```python
from build123d import *

# Parameters (mm, degrees)
SKETCH003_W          = 7
SKETCH003_H          = 3
SKETCH004_W          = 7
SKETCH004_H          = 3
SKETCH005_W          = 7
SKETCH005_H          = 3
SKETCH006_W          = 7
SKETCH006_H          = 3
POCKET_DEPTH         = 6.001
POCKET_DEPTH_BACK    = -6.001
POCKET001_DEPTH      = 6.001
POCKET001_DEPTH_BACK = -6.001
POCKET002_DEPTH      = 6.001
POCKET002_DEPTH_BACK = -6.001


with BuildPart() as part:
    # AdditivePipe: sweep along a path in Sketch
    with BuildLine(Plane.XY) as additivepipe_path:
        Line((0, 0), (0, 144))
    # Sketch002 → AdditivePipe (sweep)
    with BuildSketch(Plane.XZ):
        Polygon((-20, 6), (-20, -6), (-16, -6), (-16, -3), (-9, -3), (-9, -6), (9, -6), (9, -3), (16, -3), (16, -6), (20, -6), (20, 6), (16, 6), (16, 3), (9, 3), (9, 6), (-9, 6), (-9, 3), (-16, 3), (-16, 6), align=None)
    sweep(path=additivepipe_path.line)

    # AdditivePipe001: sweep along a path in Sketch001
    with BuildLine(Plane.XY) as additivepipe001_path:
        Line((0, 0), (0, 12))
        ThreePointArc((0, 12), (11.467071, 41.510976), (20, 72))
        ThreePointArc((20, 72), (28.532929, 102.489024), (40, 132))
        Line((40, 132), (40, 144))
    # Sketch002 → AdditivePipe001 (sweep)
    with BuildSketch(Plane.XZ):
        Polygon((-20, 6), (-20, -6), (-16, -6), (-16, -3), (-9, -3), (-9, -6), (9, -6), (9, -3), (16, -3), (16, -6), (20, -6), (20, 6), (16, 6), (16, 3), (9, 3), (9, 6), (-9, 6), (-9, 3), (-16, 3), (-16, 6), align=None)
    sweep(path=additivepipe001_path.line)

    # SubtractivePipe: sweep along a path in Sketch
    with BuildLine(Plane.XY) as subtractivepipe_path:
        Line((0, 0), (0, 144))
    # Sketch003 → SubtractivePipe (sweep, cut)
    with BuildSketch(Plane.XZ):
        with Locations((-12.5, 4.5)):
            Rectangle(SKETCH003_W, SKETCH003_H)
    sweep(path=subtractivepipe_path.line, mode=Mode.SUBTRACT)

    # SubtractivePipe001: sweep along a path in Sketch001
    with BuildLine(Plane.XY) as subtractivepipe001_path:
        Line((0, 0), (0, 12))
        ThreePointArc((0, 12), (11.467071, 41.510976), (20, 72))
        ThreePointArc((20, 72), (28.532929, 102.489024), (40, 132))
        Line((40, 132), (40, 144))
    # Sketch003 → SubtractivePipe001 (sweep, cut)
    with BuildSketch(Plane.XZ):
        with Locations((-12.5, 4.5)):
            Rectangle(SKETCH003_W, SKETCH003_H)
    sweep(path=subtractivepipe001_path.line, mode=Mode.SUBTRACT)

    # SubtractivePipe002: sweep along a path in Sketch
    with BuildLine(Plane.XY) as subtractivepipe002_path:
        Line((0, 0), (0, 144))
    # Sketch004 → SubtractivePipe002 (sweep, cut)
    with BuildSketch(Plane.XZ):
        with Locations((12.5, 4.5)):
            Rectangle(SKETCH004_W, SKETCH004_H)
    sweep(path=subtractivepipe002_path.line, mode=Mode.SUBTRACT)

    # SubtractivePipe003: sweep along a path in Sketch001
    with BuildLine(Plane.XY) as subtractivepipe003_path:
        Line((0, 0), (0, 12))
        ThreePointArc((0, 12), (11.467071, 41.510976), (20, 72))
        ThreePointArc((20, 72), (28.532929, 102.489024), (40, 132))
        Line((40, 132), (40, 144))
    # Sketch004 → SubtractivePipe003 (sweep, cut)
    with BuildSketch(Plane.XZ):
        with Locations((12.5, 4.5)):
            Rectangle(SKETCH004_W, SKETCH004_H)
    sweep(path=subtractivepipe003_path.line, mode=Mode.SUBTRACT)

    # SubtractivePipe004: sweep along a path in Sketch
    with BuildLine(Plane.XY) as subtractivepipe004_path:
        Line((0, 0), (0, 144))
    # Sketch005 → SubtractivePipe004 (sweep, cut)
    with BuildSketch(Plane.XZ):
        with Locations((-12.5, -4.5)):
            Rectangle(SKETCH005_W, SKETCH005_H)
    sweep(path=subtractivepipe004_path.line, mode=Mode.SUBTRACT)

    # SubtractivePipe005: sweep along a path in Sketch001
    with BuildLine(Plane.XY) as subtractivepipe005_path:
        Line((0, 0), (0, 12))
        ThreePointArc((0, 12), (11.467071, 41.510976), (20, 72))
        ThreePointArc((20, 72), (28.532929, 102.489024), (40, 132))
        Line((40, 132), (40, 144))
    # Sketch005 → SubtractivePipe005 (sweep, cut)
    with BuildSketch(Plane.XZ):
        with Locations((-12.5, -4.5)):
            Rectangle(SKETCH005_W, SKETCH005_H)
    sweep(path=subtractivepipe005_path.line, mode=Mode.SUBTRACT)

    # SubtractivePipe006: sweep along a path in Sketch
    with BuildLine(Plane.XY) as subtractivepipe006_path:
        Line((0, 0), (0, 144))
    # Sketch006 → SubtractivePipe006 (sweep, cut)
    with BuildSketch(Plane.XZ):
        with Locations((12.5, -4.5)):
            Rectangle(SKETCH006_W, SKETCH006_H)
    sweep(path=subtractivepipe006_path.line, mode=Mode.SUBTRACT)

    # SubtractivePipe007: sweep along a path in Sketch001
    with BuildLine(Plane.XY) as subtractivepipe007_path:
        Line((0, 0), (0, 12))
        ThreePointArc((0, 12), (11.467071, 41.510976), (20, 72))
        ThreePointArc((20, 72), (28.532929, 102.489024), (40, 132))
        Line((40, 132), (40, 144))
    # Sketch006 → SubtractivePipe007 (sweep, cut)
    with BuildSketch(Plane.XZ):
        with Locations((12.5, -4.5)):
            Rectangle(SKETCH006_W, SKETCH006_H)
    sweep(path=subtractivepipe007_path.line, mode=Mode.SUBTRACT)

    # Sketch007 → Pocket (cut, two sides)
    with BuildSketch(Plane.XY) as pocket_sk:
        with BuildLine():
            Line((-4.5, 0), (4.5, 0))
            Line((4.5, 0), (4.5, 7))
            ThreePointArc((4.5, 7), (0, 19.361903), (-4.5, 7))
            Line((-4.5, 0), (-4.5, 7))
        make_face()
    extrude(amount=-POCKET_DEPTH, mode=Mode.SUBTRACT)
    extrude(pocket_sk.sketch, amount=-POCKET_DEPTH_BACK, mode=Mode.SUBTRACT)

    # Sketch008 → Pocket001 (cut, two sides)
    with BuildSketch(Plane.XY) as pocket001_sk:
        with BuildLine():
            Line((-4.5, 144), (4.5, 144))
            Line((4.5, 144), (4.5, 137))
            ThreePointArc((-4.5, 137), (0, 124.638097), (4.5, 137))
            Line((-4.5, 144), (-4.5, 137))
        make_face()
    extrude(amount=-POCKET001_DEPTH, mode=Mode.SUBTRACT)
    extrude(pocket001_sk.sketch, amount=-POCKET001_DEPTH_BACK, mode=Mode.SUBTRACT)

    # Sketch009 → Pocket002 (cut, two sides)
    with BuildSketch(Plane.XY) as pocket002_sk:
        with BuildLine():
            Line((35.5, 144), (44.5, 144))
            Line((44.5, 144), (44.5, 137))
            ThreePointArc((35.5, 137), (40, 124.638097), (44.5, 137))
            Line((35.5, 144), (35.5, 137))
        make_face()
    extrude(amount=-POCKET002_DEPTH, mode=Mode.SUBTRACT)
    extrude(pocket002_sk.sketch, amount=-POCKET002_DEPTH_BACK, mode=Mode.SUBTRACT)


solid = part.part
```
Can you work these out from the model? Positions are in its coordinate system, mm. A direction names the side the tool comes from. Coordinates: 2 decimals unless noted, no trailing zeros. Order: outer loops, then holes, each group sorted by start corner. A loop starts at its lowest first (then second) coordinate and runs counter-clockwise, first axis right, second up.
1. I need wall thicknesses on line 1 (X direction, y = 131.5, z = -2.75); line 2 (X direction, y = 8, z = -4.75); line 3 (Z direction, x = -10.5, y = 53). Which ranges of each line are inside material? Lowest first, please.
2. If we section it at A-A (z = -1): Please give me the cut outline in (x, y).
3. If we section it at B-B (x = 22.5): Please give me the cut outline in (y, z), then the cut area to 3 significant figures.
4. If we section it at D-D (x = 0): Please give me the cut outline in (y, z), then the cut area to 3 significant figures.
5. Thinking about a two-plate mould opening in X: for faces 1 (the face through (36, 72, -6)), 2 (the face through (31, 138, 5)), which applies, +X half, -X half, draft (parallel to the pull), parting line (faces both ways), or undercut?
6. I'm going to push flat-ended pins straight in: pin 1 (6 mm diameter, centred on y = 7, z = 0.5, fed in from +X); pin 2 (1.5 mm diameter, centred on y = 52, z = -4.5, fed in from +X); pin 3 (2.5 mm diameter, centred on y = 49.5, z = 5, fed in from +X). Where does each tip first touch, or does it pass through?
7. For faces 3 (the face through (-1.73, 47.93, -4.52)), 4 (the face through (56, 138, -4)), 5 (the face through (-9, 87, -4)), 6 (the face through (23.09, 51.1, 4.48)), which set-ups out of +Z, -Z, +X, -X, +Y, -Y let a thin tool reach every point of the face, with its end or its side?
8. If we section it at C-C (y = 84): Please give me the cut outline in (x, z).
Entries:
1. line 1: x = -20 to -7, 7 to 33, 47 to 59.76
1. line 2: x = -20 to -16, -9 to -5.47, 5.47 to 9, 16 to 20
1. line 3: z = -3 to 3
2. outline: (-20, 0) - (-4.5, 0) - (-4.5, 7) arc R7 cw (long way) to (4.5, 7) - (4.5, 0) - (20, 0) - (20, 12) arc R342.46 ccw to (39.62, 75.88) arc R305.94 cw to (60, 132) - (60, 144) - (44.5, 144) - (44.5, 137) arc R7 cw (long way) to (35.5, 137) - (35.5, 144) - (4.5, 144) - (4.5, 137) arc R7 cw (long way) to (-4.5, 137) - (-4.5, 144) - (-20, 144) - close
3. outline: (18.15, -6) - (28.56, -6) - (28.56, -3) - (49.1, -3) - (49.1, -6) - (110.3, -6) - (110.3, -3) - (128.4, -3) - (128.4, -6) - (144, -6) - (144, 6) - (128.4, 6) - (128.4, 3) - (110.3, 3) - (110.3, 6) - (49.1, 6) - (49.1, 3) - (28.56, 3) - (28.56, 6) - (18.15, 6) - close
3. area: 1,280 mm2
4. outline: (19.36, -6) - (33.65, -6) - (33.65, -3) - (53.4, -3) - (53.4, -6) - (124.64, -6) - (124.64, 6) - (53.4, 6) - (53.4, 3) - (33.65, 3) - (33.65, 6) - (19.36, 6) - close
4. area: 1,140 mm2
5. face 1: draft
5. face 2: undercut
6. pin 1: stops at x = 20
6. pin 2: stops at x = 34.08
6. pin 3: stops at x = 33.52
7. face 3: -Z
7. face 4: -Z, +Y
7. face 5: -Z, +Y, -Y
7. face 6: +Z
8. outline: (-20, -6) - (-16, -6) - (-16, -3) - (-9, -3) - (-9, -6) - (7.8, -6) - (7.8, -3) - (16, -3) - (16, -6) - (31.47, -6) - (31.47, -3) - (38.06, -3) - (38.06, -6) - (41.82, -6) - (41.82, 6) - (38.06, 6) - (38.06, 3) - (31.47, 3) - (31.47, 6) - (16, 6) - (16, 3) - (7.8, 3) - (7.8, 6) - (-9, 6) - (-9, 3) - (-16, 3) - (-16, 6) - (-20, 6) - close
